```python
from build123d import *

# Parameters (mm, degrees)
BOSS_EXTRUDE1_DEPTH           = 4
DRAFT1_ANGLE                  = 45.000000004
DRAFT2_ANGLE                  = 45.000000005
F_4_0_4_DIAMETER_HOLE1_D      = 4
FILLET1_R                     = 1
FILLET2_R                     = 6.5
CSK_FOR_M3_SFHCS2_D           = 2.5
CSK_FOR_M3_SFHCS2_CSINK_D     = 4
CSK_FOR_M3_SFHCS2_CSINK_ANGLE = 90


with BuildPart() as part:
    # Sketch1 → Boss-Extrude1 (new body)
    with BuildSketch(Plane.XZ.offset(2)):
        with BuildLine():
            Line((11.124319466, 26.5), (-6.5, 26.5))
            Line((-6.5, 26.5), (-6.5, 0))
            ThreePointArc((-6.5, 0), (3e-09, -6.500000003), (6.500000005, 0))
            Line((6.500000005, 0), (6.500000005, 20.5))
            Line((6.500000005, 20.5), (13.60960084, 20.5))
            Line((13.60960084, 20.5), (13.60960084, 36.100603473))
            Line((13.60960084, 36.100603473), (11.124319466, 38.585884847))
            Line((11.124319466, 38.585884847), (11.124319466, 26.5))
        make_face()
    extrude(amount=-BOSS_EXTRUDE1_DEPTH)

    # Draft1
    draft1_faces = [part.faces().sort_by_distance(p)[0] for p in [
        (13.60960084, 0, 28.300301737),
    ]]
    draft(draft1_faces, Plane(origin=(6.500000005, 2, 20.5), x_dir=(-1, 0, 0), z_dir=(0, 0, -1)), DRAFT1_ANGLE)

    # Draft2
    draft2_faces = [part.faces().sort_by_distance(p)[0] for p in [
        (11.124319466, 0, 32.542942424),
    ]]
    draft(draft2_faces, Plane(origin=(11.124319466, 2, 26.5), x_dir=(1, 0, 0), z_dir=(0, 0, 1)), DRAFT2_ANGLE)

    # Sketch2 → Cut-Revolve1 (revolve, cut)
    with BuildSketch(Plane.XY.offset(20)):
        Polygon((0, 3.195464025), (0, -2), (6, -2), (6, -1), (5, -1), (5, 3.195464025), align=None)
    revolve(axis=Axis((0, 3.195464025, 20), (0, -1, 0)), mode=Mode.SUBTRACT)

    # Ø4.0 (4) Diameter Hole1 (through all)
    with Locations(Plane(origin=(0, 2, 0), x_dir=(1, 0, 0), z_dir=(0, 1, 0))):
        with Locations((0, 2.5)):
            Hole(F_4_0_4_DIAMETER_HOLE1_D / 2)

    # Fillet1
    fillet1_edges = [part.edges().sort_by_distance(p)[0] for p in [
        (13.60960084, 0, 20.5),
        (6.500000005, 0, 20.5),
        (11.124319466, 0, 26.5),
    ]]
    fillet(fillet1_edges, radius=FILLET1_R)

    # Fillet2
    fillet2_edges = [part.edges().sort_by_distance(p)[0] for p in [
        (-6.5, 0, 26.5),
    ]]
    fillet(fillet2_edges, radius=FILLET2_R)

    # CSK for M3 SFHCS2 (through all)
    with Locations(Plane(origin=(18.227922062, 2, 27.946748346), x_dir=(0, 0, 1), z_dir=(0, 1, 0))):
        with Locations((0, 0), (-3.535533906, -3.535533907)):
            CounterSinkHole(CSK_FOR_M3_SFHCS2_D / 2, CSK_FOR_M3_SFHCS2_CSINK_D / 2, counter_sink_angle=CSK_FOR_M3_SFHCS2_CSINK_ANGLE)


solid = part.part
```
The listing builds one solid part. Answer for the finished solid, in the listing's coordinates (mm). A direction names the side the tool comes from. Round coordinates to 2 decimals unless told otherwise and drop trailing zeros. Loops run counter-clockwise (first coordinate to the right, second up) from the corner with the lowest first, then second, coordinate; pieces in that order, holes last.
Q1. Given pin 1 Ø9.5 at (x, z) = (0, 20) entering from +Y (1 decimal); pin 2 Ø1.2 at (y, z) = (-0.5, 10.5) entering from +X, each flat-ended and moving along its own axis, determine where each tip first touches the part or whether it passes through.
Q2. For a pull along Z with two mould halves and no side action, classify faces 6 (the face through (-5.994, -1.493, 20.264)), 7 (the face through (10, 0, 20.5)), 8 (the face through (19.32, -0.03, 30.39)), 9 (the face through (19.28, -0.4, 27.27)) as released by +Z, released by -Z, zero draft, split by the parting line, or undercut.
Q3. Find the intervals of material crossed by line 1 (Z direction, x = 0, y = -1.2); line 2 (Z direction, x = 0, y = 0.2); line 3 (X direction, y = -1.15, z = 10.5), in increasing order.
Q4. Section B-B, the plane y = -1.45 is taken. Determine the outline of the cut face in (x, z), then the cut area to 3 significant figures.
Q5. Section D-D, the plane z = 16.5 is taken. Determine the outline of the cut face in (x, y).
Q6. Section C-C, the plane z = 12 is taken. Determine the outline of the cut face in (x, y).
Q7. Section A-A, the plane z = -2.5 is taken. Determine the outline of the cut face in (x, y).
Q8. Which of the six approach directions +Z, -Z, +X, -X, +Y, -Y give full straight-line access (tool end or side, diameter ignored) to faces 1 (the face through (5, 0, 26.5)), 2 (the face through (-4, -1, 24)), 3 (the face through (-0.1, 0, -6.5)), 4 (the face through (-1.08, 0.52, 15.12)), 5 (the face through (6.5, 0, 10))?
Completed:
1. pin 1: passes through
1. pin 2: stops at x = 6.5
2. face 6: undercut
2. face 7: released by -Z
2. face 8: released by +Z
2. face 9: undercut
3. line 1: z = -6.5 to -4.5, -0.5 to 14, 26 to 26.5
3. line 2: z = -6.5 to -4.5, -0.5 to 15, 25 to 26.5
3. line 3: x = -6.5 to 6.5
4. outline: (-6.5, 0) arc R6.5 ccw to (6.5, 0) - (6.5, 19.5) arc R1 cw to (7.5, 20.5) - (13.2, 20.5) arc R1 ccw to (13.9, 20.79) - (21.41, 28.3) - (17.17, 32.54) - (11.42, 26.79) arc R1 cw to (10.71, 26.5) - (0, 26.5) arc R6.5 ccw to (-6.5, 20) - close; hole circle Ø12 at (0, 20); hole circle Ø4 at (0, -2.5); hole circle Ø2.5 at (14.69, 24.41); hole circle Ø2.5 at (18.23, 27.95)
4. area: 360 mm2
5. outline: (-6.5, -2) - (-4.87, -2) - (-4.87, -1) - (-3.57, -1) - (-3.57, 2) - (-6.5, 2) - close; (3.57, -1) - (4.87, -1) - (4.87, -2) - (6.5, -2) - (6.5, 2) - (3.57, 2) - close
6. outline: (-6.5, -2) - (6.5, -2) - (6.5, 2) - (-6.5, 2) - close
7. outline: (-6, -2) - (-2, -2) - (-2, 2) - (-6, 2) - close; (2, -2) - (6, -2) - (6, 2) - (2, 2) - close
8. face 1: +Z, -X, +Y, -Y
8. face 2: -Y
8. face 3: -Z, +Y, -Y
8. face 4: +Y, -Y
8. face 5: -Z, +X, +Y, -Y
